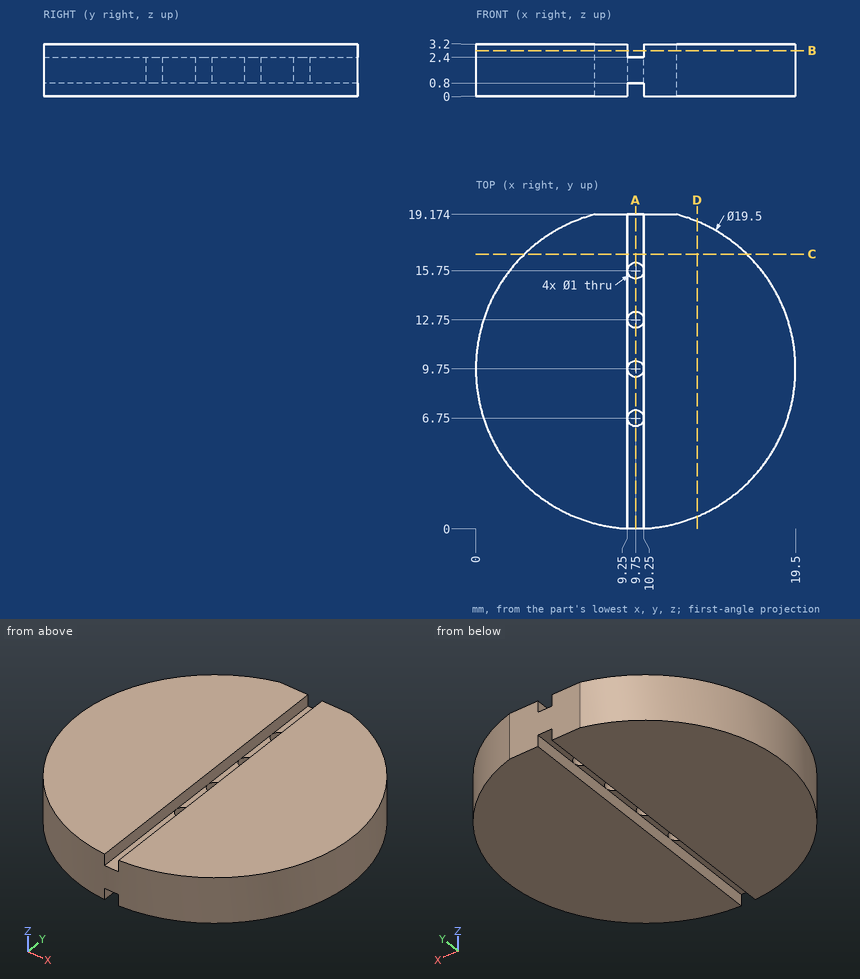
Part print with two shaded views. Sizes in mm from the minimum x, y, z corner. Round coordinates to 2 decimals unless told otherwise and drop trailing zeros. Write each loop counter-clockwise with the first axis right and the second up, starting at its lowest first coordinate (ties: lowest second). Pieces come first, ordered by that corner, then holes. Notation, with made-up numbers: (58, 60.25) - (73, 60.25) arc R15 cw to (73, 84.25) - close; hole circle Ø6 at (-34, -20.5). An arc over 180 degrees is marked (long way). Use CSV: the item, a comma, the result in double quotes.
Item 1: Slice it at C-C, the plane y = 16.75. Write the cut outline in (x, z), then the cut area to 3 significant figures.
Results list:
outline,"(2.96, 0) - (9.25, 0) - (9.25, 0.8) - (10.25, 0.8) - (10.25, 0) - (16.54, 0) - (16.54, 3.2) - (10.25, 3.2) - (10.25, 2.4) - (9.25, 2.4) - (9.25, 3.2) - (2.96, 3.2) - close"
area,"41.8 mm²"
Item 2: Slice it at A-A, the plane x = 9.75. Write the cut outline in (y, z), then the cut area to 3 significant figures.
Results list:
outline,"(0, 0.8) - (6.25, 0.8) - (6.25, 2.4) - (0, 2.4) - close; (7.25, 0.8) - (9.25, 0.8) - (9.25, 2.4) - (7.25, 2.4) - close; (10.25, 0.8) - (12.25, 0.8) - (12.25, 2.4) - (10.25, 2.4) - close; (13.25, 0.8) - (15.25, 0.8) - (15.25, 2.4) - (13.25, 2.4) - close; (16.25, 0.8) - (19.17, 0.8) - (19.17, 2.4) - (16.25, 2.4) - close"
area,"24.3 mm²"
Item 3: Slice it at B-B, the plane z = 2.8. Write the cut outline in (x, y), then the cut area to 3 significant figures.
Results list:
outline,"(7.25, 19.17) arc R9.75 ccw to (9.25, 0.01) - (9.25, 19.17) - close; (10.25, 0.01) arc R9.75 ccw to (12.25, 19.17) - (10.25, 19.17) - close"
area,"278 mm²"
Item 4: Slice it at D-D, the plane x = 13.5. Write the cut outline in (y, z), then the cut area to 3 significant figures.
Results list:
outline,"(0.75, 0) - (18.75, 0) - (18.75, 3.2) - (0.75, 3.2) - close"
area,"57.6 mm²"
Item 5: Wall check: L1, parallel to X at y = 9.75, z = 1.45; L2, parallel to Y at x = 9.75, z = 1.7; L3, parallel to X at y = 12.75, z = 1.65. Give the ranges that are in metal, low to high.
Results list:
L1,"x = 0 to 9.25, 10.25 to 19.5"
L2,"y = 0 to 6.25, 7.25 to 9.25, 10.25 to 12.25, 13.25 to 15.25, 16.25 to 19.17"
L3,"x = 0.47 to 9.25, 10.25 to 19.03"
Item 6: Flat gauge pins, fed straight in: P1, Ø1, axis at x = 8, z = 2, coming from the -Y side; P2, Ø0.6, axis at y = 10.5, z = 0.5, coming from the +X side. Where does each tip first touch, or does it go through?
Results list:
P1,"stops at y = 0.08"
P2,"stops at x = 19.49"
